Design review of the part built by this model. Coordinates are the model's own, in mm. Face numbers are marked on the shaded views. Round coordinates to 2 decimals unless told otherwise and drop trailing zeros. Loops run counter-clockwise (first coordinate to the right, second up) from the corner with the lowest first, then second, coordinate; pieces in that order, holes last. Notation, with made-up numbers: M -2.5,-5.75 L 25.5,-5.75 A19 cw 25.5,14.25 Z; hole C -23,-20.75 d11. An arc over 180 degrees is marked long. Answer as CSV lines item,"result". Start each with the question number.
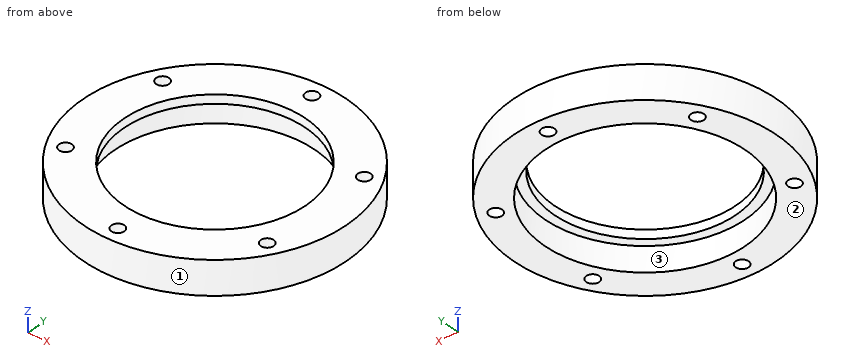
from build123d import *

# Parameters (mm, degrees)
SKETCH_1_R               = 21
SKETCH_1_R_2             = 16
EXTRUDE_1_DEPTH          = 1.97
EXTRUDE_START            = 1.4
SKETCH_2_R               = 21
SKETCH_2_R_2             = 14.5
EXTRUDE_2_DEPTH          = 1.4
HOLE_WIZARD_M2_5_1_D     = 2.05
PATTERN_CIRCULAR_1_COUNT = 6


with BuildPart() as part:
    # 草图1 → 凸台-拉伸1 (new, symmetric)
    with BuildSketch(Plane.XY):
        Circle(SKETCH_1_R)
        Circle(SKETCH_1_R_2, mode=Mode.SUBTRACT)
    extrude(amount=EXTRUDE_1_DEPTH, both=True)

    # 草图2 → 凸台-拉伸2 (add)
    with BuildSketch(Plane.XY.offset(1.97).offset(EXTRUDE_START)):
        Circle(SKETCH_2_R)
        Circle(SKETCH_2_R_2, mode=Mode.SUBTRACT)
    extrude(amount=-EXTRUDE_2_DEPTH)

    # M2.5 螺纹孔1 (through all)
    with Locations(Plane(origin=(0, 0, -1.97), x_dir=(-1, 0, 0), z_dir=(0, 0, -1))):
        with Locations((0, 18.5)):
            hole_wizard_m2_5_1 = Hole(HOLE_WIZARD_M2_5_1_D / 2)

    # 阵列(圆周)1: M2.5 螺纹孔1 ×6 about axis
    pattern_circular_1_axis = Axis((0, 0, 0), (0, 0, 1))
    for i in range(1, PATTERN_CIRCULAR_1_COUNT):
        add(hole_wizard_m2_5_1.rotate(pattern_circular_1_axis, i * 360 / PATTERN_CIRCULAR_1_COUNT), mode=Mode.SUBTRACT)


solid = part.part
Item 1: Consider section C-C, the plane z = 2.5. Write out the cut boundary in (x, y) (3 decimals), then the cut area to 3 significant figures.
Item 2: Consider section B-B, the plane y = 0. Write out the cut boundary in (x, z), then the cut area to 3 significant figures.
Item 3: Consider section A-A, the plane x = 0. Write out the cut boundary in (y, z) (3 decimals).
Item 4: Consider section D-D, the plane x = 13.5. Write out the cut boundary in (y, z).
Item 5: The part is to be moulded in two halves that separate along X. For the marked faces 1, 2 and 3, say which applies: +X half, -X half, draft (parallel to the pull), parting line (faces both ways), or undercut.
Item 6: Insertion check: pin 1 Ø3 at (x, z) = (-8, -1.5) entering from +Y; pin 2 Ø3 at (x, z) = (-2.5, 2) entering from +Y; pin 3 Ø1.5 at (y, z) = (12, 1.5) entering from +X. Each pin has a flat end and moves straight along its axis. Give the tip position at first contact, or say it passes through.
Item 7: To check wall thickness, follow line 1 (Y direction, x = 0, z = 0) (3 decimals); line 2 (Y direction, x = 0, z = 3) (3 decimals); line 3 (Y direction, x = 16, z = 2.05). State the ranges of each line that lie inside material, in increasing order.
Found:
1,outline,"C 0,0 d42; hole C -16.021,-9.25 d2.05; hole C -16.021,9.25 d2.05; hole C 0,0 d29; hole C 0,-18.5 d2.05; hole C 0,18.5 d2.05; hole C 16.021,-9.25 d2.05; hole C 16.021,9.25 d2.05"
1,area,"705 mm^2"
2,outline,"M -21,-1.97 L -16,-1.97 L -16,1.97 L -14.5,1.97 L -14.5,3.37 L -21,3.37 Z; M 14.5,1.97 L 16,1.97 L 16,-1.97 L 21,-1.97 L 21,3.37 L 14.5,3.37 Z"
2,area,"57.6 mm^2"
3,outline,"M -21,-1.97 L -19.525,-1.97 L -19.525,3.37 L -21,3.37 Z; M -17.475,-1.97 L -16,-1.97 L -16,1.97 L -14.5,1.97 L -14.5,3.37 L -17.475,3.37 Z; M 14.5,1.97 L 16,1.97 L 16,-1.97 L 17.475,-1.97 L 17.475,3.37 L 14.5,3.37 Z; M 19.525,-1.97 L 21,-1.97 L 21,3.37 L 19.525,3.37 Z"
4,outline,"M -16.09,-1.97 L -8.59,-1.97 L -8.59,1.97 L -5.29,1.97 L -5.29,3.37 L -16.09,3.37 Z; M 5.29,1.97 L 8.59,1.97 L 8.59,-1.97 L 16.09,-1.97 L 16.09,3.37 L 5.29,3.37 Z"
5,face 1,"parting line"
5,face 2,"draft"
5,face 3,"undercut"
6,pin 1,"stops at y = 19.97"
6,pin 2,"stops at y = 20.98"
6,pin 3,"stops at x = 17.73"
7,line 1,"y = -21 to -19.525, -17.475 to -16, 16 to 17.475, 19.525 to 21"
7,line 2,"y = -21 to -19.525, -17.475 to -14.5, 14.5 to 17.475, 19.525 to 21"
7,line 3,"y = -13.6 to -10.27, -8.23 to 8.23, 10.27 to 13.6"
